The model under review builds one solid part; all positions refer to its coordinate system, in mm. A direction names the side the tool comes from. Give positions to 0.01 mm unless a question says otherwise; leave off trailing zeros. Write each loop counter-clockwise with the first axis right and the second up, starting at its lowest first coordinate (ties: lowest second). Pieces come first, ordered by that corner, then holes. Notation, with made-up numbers: (13, 72) - (19, 72) arc R26 ccw to (19, 99) - close; hole circle Ø11 at (-32.75, 65.5). An arc over 180 degrees is marked (long way). Write item = value, one per line.
```python
from build123d import *

# Parameters (mm, degrees)
F_0030_CYLINDER_SKETCH_R    = 3.25
F_0030_CYLINDER_DEPTH       = 2.5
F_0031_FILLET_R             = 0.625
F_0032_EXTRUDE_DEPTH        = 1.385
F_0032_EXTRUDE_ROTATE_ANGLE = 120
F_0035_CYLINDER_SKETCH_R    = 1.2
F_0035_CYLINDER_DEPTH       = 11.7
F_0036_CONE_ROTATE_ANGLE    = 90


with BuildPart() as part:
    # 0030_cylinder_Sketch → 0030_cylinder (new body)
    with BuildSketch(Plane.XY):
        Circle(F_0030_CYLINDER_SKETCH_R)
    extrude(amount=F_0030_CYLINDER_DEPTH)

    # 0031_fillet
    f_0031_fillet_edges = [part.edges().sort_by_distance(p)[0] for p in [
        (-3.25, 0, 2.5),
    ]]
    fillet(f_0031_fillet_edges, radius=F_0031_FILLET_R)


with BuildPart() as body_2:
    # 0032_extrude_Sketch → 0032_extrude (new body)
    with BuildSketch(Plane.XY):
        Polygon((0, 0), (1.154700538, 0), (1.732050808, 1), (1.154700538, 2), (0, 2), (-0.577350269, 1), align=None)
    extrude(amount=F_0032_EXTRUDE_DEPTH)


with BuildPart() as body_2_1:
    # 0032_extrude_Rotate: read off the stored shape, not the designer's step
    # 0032_extrude_Rotate: moved
    add(body_2.part.rotate(Axis((0, 0, 0), (0, 0, 1)), F_0032_EXTRUDE_ROTATE_ANGLE))


with BuildPart() as body_2_2:
    # 0032_extrude_Translate: moved
    add(body_2_1.part.moved(Location((1.154700538, 0, 1.125))))


with BuildPart() as part_1:
    add(part.part)

    # 0034_sub: cut body 2
    add(body_2_2.part, mode=Mode.SUBTRACT)


with BuildPart() as body_2_2_1:
    # 0035_cylinder_Sketch → 0035_cylinder (new body)
    with BuildSketch(Plane.XY):
        Circle(F_0035_CYLINDER_SKETCH_R)
    extrude(amount=F_0035_CYLINDER_DEPTH)


with BuildPart() as body_2_2_2:
    # 0035_cylinder_Translate: moved
    add(body_2_2_1.part.moved(Location((0, 0, -11.7))))


with BuildPart() as body_3:
    # 0036_cone_Sketch → 0036_cone (revolve)
    with BuildSketch(Plane.XY, mode=Mode.PRIVATE) as f_0036_cone_sk:
        Polygon((0, 0), (1.2, 0), (0.9, 0.3), (0, 0.3), align=None)
    revolve(f_0036_cone_sk.sketch.rotate(Axis((0, -100, 0), (0, 1, 0)), 90), axis=Axis((0, -100, 0), (0, 1, 0)))


with BuildPart() as body_3_1:
    # 0036_cone_Rotate: moved
    add(body_3.part.rotate(Axis((0, 0, 0), (1, 0, 0)), F_0036_CONE_ROTATE_ANGLE))


with BuildPart() as body_3_2:
    # 0036_cone_Translate: moved
    add(body_3_1.part.moved(Location((0, 0, -12))))


with BuildPart() as body_2_2_3:
    add(body_2_2_2.part)

    # 0038_add: union body 3
    add(body_3_2.part)


with BuildPart() as part_2:
    add(part_1.part)

    # 0039_add: union body 2 2
    add(body_2_2_3.part)


solid = part_2.part
```
1. Machinability: for faces 1 (the flat face through (-0.86, 0.51, 1.8)), 2 (the flat face through (1.4, 0, 0)), 3 (the flat face through (1, -1, 2.5)), which of the approach directions +Z, -Z, +X, -X, +Y, -Y give a long, thin tool a straight path to every point of the face, cutting with its end or side? Answer none if there is none.
Findings below:
face_1 = +Z
face_2 = -Z
face_3 = +Z, +X, -X, +Y, -Y
2. Take a section at B-B on z = -1. Give the boundary of the cut face in (x, y).
Findings below:
outline = circle Ø2.4 at (0, 0)
3. Take a section at A-A on x = 0. Give the boundary of the cut face in (y, z) (3 decimals), and give its area (3 significant figures).
Findings below:
outline = (-3.25, 0) - (-1.2, 0) - (-1.2, -11.7) - (-0.9, -11.7) - (-1.2, -12) - (1.2, -12) - (0.9, -11.7) - (1.2, -11.7) - (1.2, 0) - (3.25, 0) - (3.25, 1.875) arc R0.625 ccw to (2.625, 2.5) - (1, 2.5) - (1, 1.125) - (-1, 1.125) - (-1, 2.5) - (-2.625, 2.5) arc R0.625 ccw to (-3.25, 1.875) - close
area = 42.0 mm²
4. For line 1 (Z direction, x = -1.25, y = -0.25); line 2 (X direction, y = 0.5, z = -4.75); line 3 (X direction, y = -0.75, z = 1.5), list the stretches that pass through material, from the lowest coordinate up. Write a range as from..to.
Findings below:
line_1 = 0..2.5
line_2 = -1.09..1.09
line_3 = -3.16..-0.72, 0.72..3.16
5. Insertion check: P1, Ø0.6, axis at x = 0, y = 0, coming from the +Z side (3 decimals); P2, Ø1, axis at x = 2.5, y = 2.5, coming from the -Z side; P3, Ø1.5, axis at y = 0, z = -5, coming from the -X side; P4, Ø1.3, axis at x = 0, z = 2, coming from the +Y side. Each pin has a flat end and moves straight along its axis. Give the tip position at first contact, or say it passes through.
Findings below:
P1 = 1.125
P2 = 0
P3 = -1.2
P4 = 3.25
6. Take a section at C-C on z = 0.5. Give the boundary of the cut face in (x, y).
Findings below:
outline = circle Ø6.5 at (0, 0)
